Part print with two shaded views. Sizes in mm from the minimum x, y, z corner. A direction names the side the tool comes from. Coordinates: 2 decimals unless noted, no trailing zeros. Write each loop counter-clockwise with the first axis right and the second up, starting at its lowest first coordinate (ties: lowest second). Pieces come first, ordered by that corner, then holes. Notation, with made-up numbers: M 40.5,-40 L 83.5,-40 A29 ccw 83.5,-2 Z; hole C 65.5,88.5 d7. An arc over 180 degrees is marked long. One line per question, with ' | ' between items. Start each with the question number.
(1) Wall check: probe 1 along X at (y, z) = (3, 25) (1 decimal); probe 2 along Z at (x, y) = (70.5, 41); probe 3 along X at (y, z) = (23, 72.5). Give the ranges that are in metal, low to high.
(2) Flat gauge pins, fed straight in: pin 1 Ø4 at (y, z) = (16.5, 52) entering from +X (1 decimal); pin 2 Ø6 at (y, z) = (31.5, 146.5) entering from +X; pin 3 Ø3 at (x, y) = (13.5, 4) entering from -Z (3 decimals); pin 4 Ø7.5 at (x, z) = (9.525, 88.9) entering from +Y. Where does each tip first touch, or does it go through?
(3) Cut at C-C (y = 55.5). Write the cut outline in (x, z), plus the area to 3 significant figures.
(4) Cut at D-D (z = 158.5). Write the cut outline in (x, y) (1 decimal).
(5) Two-plate mould, pull along Y, no slides. Class the marked faces 5, 6 and 7: +Y half, -Y half, draft (parallel to the pull), parting line (faces both ways), or undercut.
(6) Cut at B-B (x = 56). Write the cut outline in (y, z).
(7) Tool access for the marked faces 1, 2, 3 and 4: list every direction of +Z, -Z, +X, -X, +Y, -Y with a clear straight run to the whole face (end or side of a thin tool).
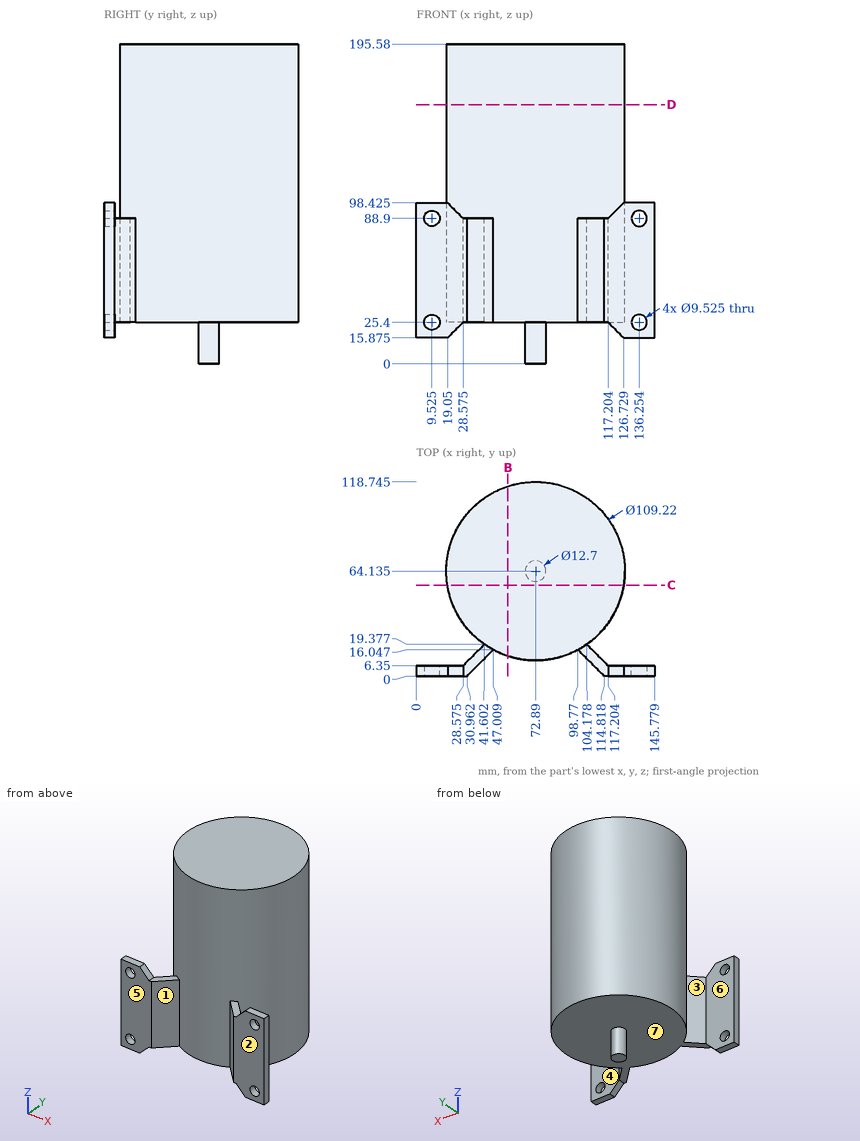
Filled in:
1) probe 1: 0 to 4.8, 14.3 to 28.2, 117.6 to 131.5, 141 to 145.8 | probe 2: 25.4 to 195.58 | probe 3: 36.97 to 108.81
2) pin 1: x = 109.1 | pin 2: x = 118.76 | pin 3: z = 15.875 | pin 4: through
3) outline: M 18.97,25.4 L 126.81,25.4 L 126.81,195.58 L 18.97,195.58 Z | area: 18,400 mm²
4) outline: C 72.9,64.1 d109.2
5) face 5: -Y half | face 6: undercut | face 7: draft
6) outline: M 12.2,25.4 L 116.07,25.4 L 116.07,195.58 L 12.2,195.58 Z
7) face 1: +Z, -Z, -Y | face 2: +Z, -Z, +X, -X, -Y | face 3: +Z, -Z, -X | face 4: +Z, -Z, +X
